Autodesk Inventor part; units mm, degrees
ref_plane "YZ Plane" through (0, 0, 0) normal (1, 0, 0) x (0, 1, 0)
ref_plane "XZ Plane" through (0, 0, 0) normal (0, 1, 0) x (-1, 0, 0)
ref_plane "XY Plane" through (0, 0, 0) normal (0, 0, 1) x (1, 0, 0)
sketch "Sketch1" plane through (0, 0, 0) normal (0, 0, 1) x (1, 0, 0)
  line L0 (797.4752, 0) -> (797.4752, -661.8669) construction
  line L1 (797.4752, -661.8669) -> (0, -661.8669)
  line L2 (751.1573, -579.8638) -> (684.3931, -661.8669) construction
  ellipse E0 centre (-10250, 795.2799) end of major axis (-10250.7907, -13633.3868) minor radius 11053 (753.0187, -574.9033) -> (782.4805, -83.0791) ccw construction
  line L3 (797.4752, 0) -> (762.6352, -581.6047)
  line L4 (697.2883, -661.8669) -> (797.4752, -538.8126)
  line L5 (753.0187, -574.9033) -> (763.0008, -575.5013) construction
  line L6 (782.4805, -83.0791) -> (792.4626, -83.6771) construction
  line L7 (0, -661.8669) -> (0, 0)
  line L8 (0, 0) -> (797.4752, 0)
  dimension "d3" = 10
  dimension "d4" = 10
  dimension "d5" = 10
extrude "Plate1" add sketch "Sketch1" along normal blind 2
mirror "Mirror1" about plane through (0, 0, 0) normal (1, 0, 0)
sketch "Sketch2" plane through (0, 0, 2) normal (0, 0, 1) x (1, 0, 0)
  line L0 (-55, -611.8669) -> (-55, -599.8669) construction
  line L1 (-55, -599.8669) -> (55, -599.8669) construction
  line L2 (55, -599.8669) -> (55, -611.8669) construction
  line L3 (55, -611.8669) -> (-55, -611.8669) construction
  line L4 (-697.2883, -661.8669) -> (697.2883, -661.8669)
  point P0 (0, 0)
  point P1 (0, -611.8669)
  point P2 (0, -661.8669)
  dimension "d6" = 12
  dimension "d7" = 110
  dimension "d8" = 50
mark "Mark1"
equation "\"d2\" = Thickness"
equation "\"BendReliefWidth\" = Thickness"
equation "\"BendReliefDepth\" = 0.5 * Thickness"
equation "\"CornerReliefSize\" = 4 * Thickness"
equation "\"MinimumRemnant\" = 2 * Thickness"
equation "\"TransitionRadius\" = BendRadius"
equation "\"JacobiRadiusSize\" = BendRadius"
equation "\"GapSize\" = Thickness"
properties part number "MSC 075 face 2" material "AISI304"
The listing builds one solid part. Answer for the finished solid, in the listing's coordinates (mm). Round coordinates to 2 decimals unless told otherwise and drop trailing zeros. Write each loop counter-clockwise with the first axis right and the second up, starting at its lowest first coordinate (ties: lowest second). Pieces come first, ordered by that corner, then holes. Notation, with made-up numbers: M 81.25,12.5 L 119.25,12.5 A15 ccw 119.25,39.5 Z; hole C -40,-36 d7. An arc over 180 degrees is marked long. Write each question's results on one line, items separated by ' | '. Start each with the question number.
Item 1: Find section B-B on z = 1.3. Write down the section's boundary in (x, y).
Item 2: Find section C-C on y = -451.5. Write down the section's boundary in (x, z).
Item 3: Straight lines are drawn through the part: probe 1 along X at (y, z) = (-221.5, 0.8); probe 2 along X at (y, z) = (-188, 0.7). For each, find the intervals that lie inside material, in ascending order.
Item 4: Find section A-A on y = -322.5. Write down the section's boundary in (x, z), and give its area (3 significant figures).
Answer block:
1) outline: M -797.48,0 L -762.64,-581.6 L -697.29,-661.87 L 697.29,-661.87 L 762.64,-581.6 L 797.48,0 Z
2) outline: M -770.43,0 L 770.43,0 L 770.43,2 L -770.43,2 Z
3) probe 1: x = -784.21 to 784.21 | probe 2: x = -786.21 to 786.21
4) outline: M -778.16,0 L 778.16,0 L 778.16,2 L -778.16,2 Z | area: 3,110 mm²
